from build123d import *

# Parameters (mm, degrees)
SKETCH1_R           = 2.5
SKETCH1_R_2         = 1.4
BOSS_EXTRUDE1_DEPTH = 7
SKETCH2_W           = 0.9
SKETCH2_H           = 6.1
BOSS_EXTRUDE2_DEPTH = 20
CUT_EXTRUDE1_REACH  = 50.836
SKETCH3_R           = 2.5
CUT_EXTRUDE2_START  = -7
CUT_EXTRUDE2_DEPTH  = 7
FILLET1_R           = 3


with BuildPart() as part:
    # Sketch1 → Boss-Extrude1 (new body)
    with BuildSketch(Plane.XY):
        with BuildLine():
            Line((3, 0), (17, 0))
            ThreePointArc((17, 0), (19.121320344, 0.878679656), (20, 3))
            Line((20, 3), (20, 41))
            ThreePointArc((20, 41), (19.121320344, 43.121320344), (17, 44))
            Line((17, 44), (3, 44))
            ThreePointArc((3, 44), (0.878679656, 43.121320344), (0, 41))
            Line((0, 41), (0, 3))
            ThreePointArc((0, 3), (0.878679656, 0.878679656), (3, 0))
        make_face()
        with Locations((10, 35)):
            Circle(SKETCH1_R, mode=Mode.SUBTRACT)
        with Locations((10, 5.4)):
            Circle(SKETCH1_R_2, mode=Mode.SUBTRACT)
        with Locations((10, 15)):
            Circle(SKETCH1_R_2, mode=Mode.SUBTRACT)
    extrude(amount=BOSS_EXTRUDE1_DEPTH)

    # Sketch2 → Boss-Extrude2 (add)
    with BuildSketch(Plane(origin=(20, 0, 0), x_dir=(0, 0, -1), z_dir=(1, 0, 0))):
        with Locations((0.45, 35)):
            Rectangle(SKETCH2_W, SKETCH2_H)
    extrude(amount=-BOSS_EXTRUDE2_DEPTH)

    # Sketch3 → Cut-Extrude1 (cut, up to next)
    with BuildSketch(Plane.XY, mode=Mode.PRIVATE) as cut_extrude1_sk1:
        with Locations((10, 35)):
            Circle(SKETCH3_R)
    cut_extrude1_tool1 = extrude(cut_extrude1_sk1.sketch, amount=-CUT_EXTRUDE1_REACH, mode=Mode.PRIVATE) & part.part
    add(cut_extrude1_tool1.solids().sort_by_distance((10, 35, 0))[0], mode=Mode.SUBTRACT)

    # Sketch4 → Cut-Extrude2 (cut)
    with BuildSketch(Plane.XY.offset(7).offset(CUT_EXTRUDE2_START)):
        with BuildLine():
            Line((0, 28), (4, 24))
            Line((4, 24), (4, 0))
            Line((4, 0), (3, 0))
            ThreePointArc((3, 0), (0.878679656, 0.878679656), (0, 3))
            Line((0, 3), (0, 28))
        make_face()
    extrude(amount=CUT_EXTRUDE2_DEPTH, mode=Mode.SUBTRACT)

    # Fillet1
    fillet1_edges = [part.edges().sort_by_distance(p)[0] for p in [
        (0, 28, 3.5),
        (4, 24, 3.5),
        (4, 0, 3.5),
    ]]
    fillet(fillet1_edges, radius=FILLET1_R)


solid = part.part
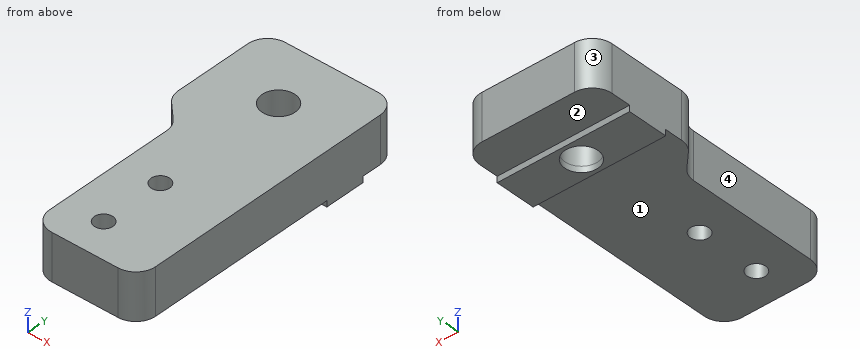
Check sheet for the modelled part. Datum: model origin and axes. Units: mm. Face numbers are marked on the shaded views. A direction names the side the tool comes from. Round coordinates to 2 decimals unless told otherwise and drop trailing zeros. Loops run counter-clockwise (first coordinate to the right, second up) from the corner with the lowest first, then second, coordinate; pieces in that order, holes last. Notation, with made-up numbers: (-28, 29) - (29, 29) arc R18 ccw to (29, 36) - close; hole circle Ø9 at (-13, 35.25). An arc over 180 degrees is marked (long way). Answer as CSV lines item,"result". Start each with the question number.
Item 1: Section check A-A (y = 35). Record the boundary of the cut face in (x, z).
Item 2: Depth check by flat-ended pin: P1, Ø2, axis at x = 10, y = 15, coming from the -Z side; P2, Ø3.5, axis at y = 14, z = 3.5, coming from the -X side; P3, Ø6, axis at x = 15, y = 8, coming from the -Z side. Enter the tip coordinate at first touch or a pass-through.
Item 3: Section check C-C (z = 1.5). Record the boundary of the cut face in (x, y).
Item 4: Scan lines: line 1 (Y direction, x = 10, z = 3.75); line 2 (Y direction, x = 10, z = -0.5); line 3 (Y direction, x = 10.5, z = 2.5). Record each from-to range of solid material in increasing order. Write a range as [from, to].
Item 5: Section check B-B (x = 10). Record the boundary of the cut face in (y, z), and give its area (3 significant figures).
Item 6: Set-up check for the marked faces 1, 2, 3 and 4: record each of +Z, -Z, +X, -X, +Y, -Y from which the full face is reachable in a straight line by a thin tool's end or side.
Item 7: Section check D-D (y = 5.4). Record the boundary of the cut face in (x, z).
Report:
1,outline,"(0, -0.9) - (7.5, -0.9) - (7.5, 7) - (0, 7) - close; (12.5, -0.9) - (20, -0.9) - (20, 7) - (12.5, 7) - close"
2,P1,"passes through"
2,P2,"stops at x = 4"
2,P3,"stops at z = 0"
3,outline,"(0, 29.24) arc R3 ccw to (0.88, 27.12) - (3.12, 24.88) arc R3 cw to (4, 22.76) - (4, 3) arc R3 ccw to (7, 0) - (17, 0) arc R3 ccw to (20, 3) - (20, 41) arc R3 ccw to (17, 44) - (3, 44) arc R3 ccw to (0, 41) - close; hole circle Ø5 at (10, 35); hole circle Ø2.8 at (10, 5.4); hole circle Ø2.8 at (10, 15)"
4,line 1,"y = [0, 4], [6.8, 13.6], [16.4, 32.5], [37.5, 44]"
4,line 2,"y = [31.95, 32.5], [37.5, 38.05]"
4,line 3,"y = [0, 4.09], [6.71, 13.69], [16.31, 32.55], [37.45, 44]"
5,outline,"(0, 0) - (4, 0) - (4, 7) - (0, 7) - close; (6.8, 0) - (13.6, 0) - (13.6, 7) - (6.8, 7) - close; (16.4, 0) - (31.95, 0) - (31.95, -0.9) - (32.5, -0.9) - (32.5, 7) - (16.4, 7) - close; (37.5, -0.9) - (38.05, -0.9) - (38.05, 0) - (44, 0) - (44, 7) - (37.5, 7) - close"
5,area,"235 mm2"
6,face 1,"-Z, +X, -X, -Y"
6,face 2,"-Z, +X, -X, +Y"
6,face 3,"+Z, -Z, -X, +Y"
6,face 4,"+Z, -Z, -X, -Y"
7,outline,"(4, 0) - (8.6, 0) - (8.6, 7) - (4, 7) - close; (11.4, 0) - (20, 0) - (20, 7) - (11.4, 7) - close"
